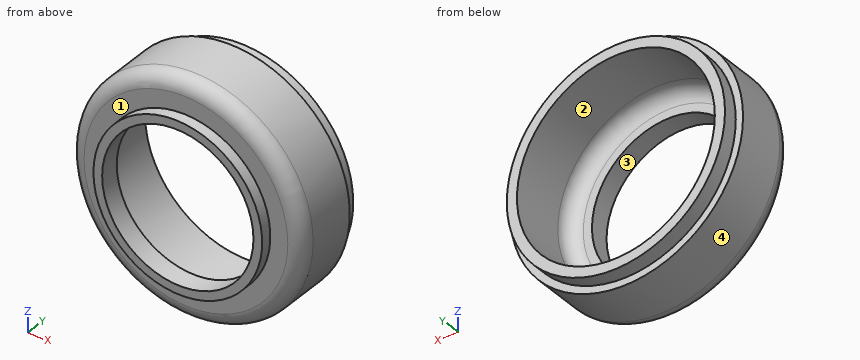
from build123d import *


with BuildPart() as part:
    # Sketch1 → Revolve1 (revolve)
    with BuildSketch(Plane.XY):
        with BuildLine():
            Line((-40, 8.79698141), (-40, -8.20301859))
            ThreePointArc((-40, -8.20301859), (-38.535533906, -11.738552496), (-35, -13.20301859))
            Line((-35, -13.20301859), (-29, -13.20301859))
            Line((-29, -13.20301859), (-29, -16.980259628))
            Line((-29, -16.980259628), (-26, -16.980259628))
            Line((-26, -16.980259628), (-26, -10.20301859))
            Line((-26, -10.20301859), (-29, -10.20301859))
            ThreePointArc((-29, -10.20301859), (-32.535533906, -8.738552496), (-34, -5.20301859))
            Line((-34, -5.20301859), (-34, 13.79698141))
            Line((-34, 13.79698141), (-37.5, 13.79698141))
            Line((-37.5, 13.79698141), (-37.5, 8.79698141))
            Line((-37.5, 8.79698141), (-40, 8.79698141))
        make_face()
    revolve(axis=Axis((0, 133.043372469, 0), (0, -1, 0)))


solid = part.part
Verification items for the finished model (mm, model axes). Face numbers are marked on the shaded views. Give positions to 0.01 mm unless a question says otherwise; leave off trailing zeros. Loops run counter-clockwise (first coordinate to the right, second up) from the corner with the lowest first, then second, coordinate; pieces in that order, holes last.
1) Depth check by flat-ended pin: pin 1 Ø10 at (y, z) = (-5.5, 28.5) entering from +X; pin 2 Ø6 at (y, z) = (2.5, 31.5) entering from +X; pin 3 Ø2 at (x, y) = (-22, 8) entering from +Z. Enter the tip coordinate at first touch or a pass-through.
2) Sectioned sample at B-B, the plane z = 0. Enter the section's corners in (x, y).
3) Sectioned sample at A-A, the plane x = 0. Enter the section's corners in (y, z), then the cut area to 3 significant figures.
4) Draft check along Z on the marked faces 1, 2, 3 and 4. Enter one of: pulls with the +Z half, pulls with the -Z half, needs draft (parallel to the pull), parting line crosses it, or undercut.
5) Sectioned sample at C-C, the plane y = 3. Enter the section's corners in (x, z), then the cut area to 3 significant figures.
6) Thickness scan on line 1 along X through (y, z) = (-15, 0); line 2 along X through (y, z) = (9, 1); line 3 along Z through (x, y) = (0, 0.5). Record the ranges inside material, lowest first.
7) Sectioned sample at D-D, the plane y = 12. Enter the section's corners in (x, z).
Answers:
1. pin 1: stops at x = 32.37
1. pin 2: stops at x = 28.07
1. pin 3: stops at z = 34.04
2. outline: (-40, -8.2) arc R5 ccw to (-35, -13.2) - (-29, -13.2) - (-29, -16.98) - (-26, -16.98) - (-26, -10.2) - (-29, -10.2) arc R5 cw to (-34, -5.2) - (-34, 13.8) - (-37.5, 13.8) - (-37.5, 8.8) - (-40, 8.8) - close; (26, -16.98) - (29, -16.98) - (29, -13.2) - (35, -13.2) arc R5 ccw to (40, -8.2) - (40, 8.8) - (37.5, 8.8) - (37.5, 13.8) - (34, 13.8) - (34, -5.2) arc R5 cw to (29, -10.2) - (26, -10.2) - close
3. outline: (-16.98, -29) - (-13.2, -29) - (-13.2, -35) arc R5 ccw to (-8.2, -40) - (8.8, -40) - (8.8, -37.5) - (13.8, -37.5) - (13.8, -34) - (-5.2, -34) arc R5 cw to (-10.2, -29) - (-10.2, -26) - (-16.98, -26) - close; (-16.98, 26) - (-10.2, 26) - (-10.2, 29) arc R5 cw to (-5.2, 34) - (13.8, 34) - (13.8, 37.5) - (8.8, 37.5) - (8.8, 40) - (-8.2, 40) arc R5 ccw to (-13.2, 35) - (-13.2, 29) - (-16.98, 29) - close
3. area: 370 mm2
4. face 1: needs draft
4. face 2: undercut
4. face 3: undercut
4. face 4: parting line crosses it
5. outline: circle Ø80 at (0, 0); hole circle Ø68 at (0, 0)
5. area: 1,390 mm2
6. line 1: x = -29 to -26, 26 to 29
6. line 2: x = -37.49 to -33.99, 33.99 to 37.49
6. line 3: z = -40 to -34, 34 to 40
7. outline: circle Ø75 at (0, 0); hole circle Ø68 at (0, 0)
